```python
from build123d import *

# Parameters (mm, degrees)
SKETCH1_W               = 104
SKETCH1_H               = 74
BOSS_EXTRUDE1_DEPTH     = 1
BOSS_EXTRUDE2_DEPTH     = 3
BOSS_EXTRUDE3_DEPTH     = 28
SKETCH3_W               = 104
SKETCH3_H               = 4
BOSS_EXTRUDE4_DEPTH     = 2
CUT_EXTRUDE1_DEPTH      = 11
CUT_EXTRUDE1_DEPTH_BACK = 11
CUT_EXTRUDE1_START      = -52
SKETCH5_W               = 104
SKETCH5_H               = 5
BOSS_EXTRUDE6_DEPTH     = 2
CUT_EXTRUDE2_START      = -32
CUT_EXTRUDE2_DEPTH      = 11
CUT_EXTRUDE3_START      = -83
CUT_EXTRUDE3_DEPTH      = 11
CHAMFER2_SIZE           = 1


with BuildPart() as part:
    # Sketch1 → Boss-Extrude1 (new body)
    with BuildSketch(Plane.XY):
        with Locations((50, 37)):
            Rectangle(SKETCH1_W, SKETCH1_H)
    extrude(amount=BOSS_EXTRUDE1_DEPTH)

    # Sketch1<3> → Boss-Extrude2 (add)
    with BuildSketch(Plane.XY):
        Polygon((-2, 74), (-2, 0), (0, 0), (0, 72), (100, 72), (100, 0), (102, 0), (102, 74), align=None)
    extrude(amount=-BOSS_EXTRUDE2_DEPTH)

    # Sketch2 → Boss-Extrude3 (add)
    with BuildSketch(Plane(origin=(0, 0, -3), x_dir=(-1, 0, 0), z_dir=(0, 0, -1))):
        Polygon((-102, 74), (2, 74), (2, 70), (0, 70), (0, 72), (-100, 72), (-100, 70), (-102, 70), align=None)
    extrude(amount=BOSS_EXTRUDE3_DEPTH)

    # Sketch3 → Boss-Extrude4 (add)
    with BuildSketch(Plane.XZ):
        with Locations((50, -1)):
            Rectangle(SKETCH3_W, SKETCH3_H)
    extrude(amount=BOSS_EXTRUDE4_DEPTH)

    # Sketch4 → Cut-Extrude1 (cut, two sides: drawn at the far end of the back side and taken through both)
    with BuildSketch(Plane.ZY.offset(2).offset(CUT_EXTRUDE1_START - CUT_EXTRUDE1_DEPTH_BACK)):
        with BuildLine():
            Line((0.2, 0), (-2.2, 0))
            ThreePointArc((-2.2, 0), (-1, -1.2), (0.2, 0))
        make_face()
    extrude(amount=CUT_EXTRUDE1_DEPTH + CUT_EXTRUDE1_DEPTH_BACK, mode=Mode.SUBTRACT)

    # Sketch5 → Boss-Extrude6 (add)
    with BuildSketch(Plane(origin=(0, 0, -31), x_dir=(-1, 0, 0), z_dir=(0, 0, -1))):
        with Locations((-50, 71.5)):
            Rectangle(SKETCH5_W, SKETCH5_H)
    extrude(amount=BOSS_EXTRUDE6_DEPTH)

    # Sketch6 → Cut-Extrude2 (cut)
    with BuildSketch(Plane.ZY.offset(2).offset(CUT_EXTRUDE2_START)):
        with BuildLine():
            ThreePointArc((-31, 72.2), (-32.2, 71), (-31, 69.8))
            Line((-31, 69.8), (-31, 72.2))
        make_face()
    extrude(amount=CUT_EXTRUDE2_DEPTH, mode=Mode.SUBTRACT)

    # Sketch6<3> → Cut-Extrude3 (cut)
    with BuildSketch(Plane.ZY.offset(2).offset(CUT_EXTRUDE3_START)):
        with BuildLine():
            ThreePointArc((-31, 72.2), (-32.2, 71), (-31, 69.8))
            Line((-31, 69.8), (-31, 72.2))
        make_face()
    extrude(amount=CUT_EXTRUDE3_DEPTH, mode=Mode.SUBTRACT)

    # Chamfer2
    chamfer2_edges = [part.edges().sort_by_distance(p)[0] for p in [
        (102, 36, 1),
        (50, 74, 1),
        (-2, 36, 1),
        (50, -2, 1),
        (50, 74, -33),
        (-2, 74, -16),
        (102, 74, -16),
    ]]
    chamfer(chamfer2_edges, length=CHAMFER2_SIZE)


solid = part.part
```
Input: part model. Units: mm. Frame: model coordinates. A direction names the side the tool comes from. Coordinates: 2 decimals unless noted, no trailing zeros. Loops run counter-clockwise (first coordinate to the right, second up) from the corner with the lowest first, then second, coordinate; pieces in that order, holes last.
Q1. Contact query for flat-ended pins moving along their axis: pin 1 (12 mm diameter, centred on x = 27.5, y = 32, fed in from -Z); pin 2 (10 mm diameter, centred on y = 34.5, z = -12, fed in from -X); pin 3 (2 mm diameter, centred on x = 73.5, z = -18.5, fed in from -Y); pin 4 (1 mm diameter, centred on x = 63, z = -32, fed in from -Y). Output: stop coordinate, or through.
Results are:
pin 1: stops at z = 0
pin 2: passes through
pin 3: stops at y = 72
pin 4: stops at y = 69
Q2. Section A-A, the plane z = -8. Return the cut outline in (x, y), and give its area (3 significant figures).
Results are:
outline: (-2, 70) - (0, 70) - (0, 72) - (100, 72) - (100, 70) - (102, 70) - (102, 73) - (101, 74) - (-1, 74) - (-2, 73) - close
area: 215 mm2
Q3. Mould query, pull axis Z, two halves, no side actions, for faces 4 (the flat face through (51, 74, -16)), 5 (the cylindrical face through (50.2, -1.2, -1)), 6 (the flat face through (51, 71, -33)), 7 (the flat face through (-1, 70, -17)). Classes: +Z half, -Z half, draft (parallel to the pull), parting line (faces both ways), or undercut.
Results are:
face 4: draft
face 5: undercut
face 6: -Z half
face 7: undercut
Q4. Section C-C, the plane y = 28.5. Return the cut outline in (x, z), and give its area (3 significant figures).
Results are:
outline: (-2, -3) - (0, -3) - (0, 0) - (100, 0) - (100, -3) - (102, -3) - (102, 0) - (101, 1) - (-1, 1) - (-2, 0) - close
area: 115 mm2
Q5. Line query: line 1 along Y through (x, z) = (89.5, -25); line 2 along Z through (x, y) = (73, 26.5). Output: solid intervals per line, ascending.
Results are:
line 1: y = 72 to 74
line 2: z = 0 to 1
Q6. Set-up query: faces 1 (the flat face through (101, 70, -17)), 2 (the flat face through (0, 41.2, -2.8)), 3 (the flat face through (51, 69, -32)). Return all of +Z, -Z, +X, -X, +Y, -Y with unobstructed straight access to the full face (end or side cutting, diameter ignored); none if empty.
Results are:
face 1: +X, -X, -Y
face 2: none
face 3: -Z, +X, -X, -Y
Q7. Section B-B, the plane x = 32. Return the cut outline in (y, z), and give its area (4 significant figures).
Results are:
outline: (-2, -3) - (0, -3) - (0, 0) - (72, 0) - (72, -31) - (69, -31) - (69, -33) - (73, -33) - (74, -32) - (74, 0) - (73, 1) - (-1, 1) - (-2, 0) - close
area: 152.5 mm2
